The listing builds one solid part. Answer for the finished solid, in the listing's coordinates (mm). A direction names the side the tool comes from. Round coordinates to 2 decimals unless told otherwise and drop trailing zeros. Write each loop counter-clockwise with the first axis right and the second up, starting at its lowest first coordinate (ties: lowest second). Pieces come first, ordered by that corner, then holes.
Item 1: A tool of negligible diameter and unlimited length cuts with its end or side. For faces 1 (the face through (-9, -0.5, -5)), 2 (the face through (-4.06, 31.5, -4.42)), from which of +Z, -Z, +X, -X, +Y, -Y can it reach the whole face along a straight path? Write none if from no direction.
Item 2: Find section C-C on y = 7. Give the vertices of the cut face in (x, z), then the cut area to 3 significant figures.
Item 3: Find the intervals of material crossed by probe 1 along Y at (x, z) = (10.25, -8.5); probe 2 along X at (y, z) = (9, 1.5); probe 3 along Z at (x, y) = (4.75, 16), in increasing order.
Item 4: Find section A-A on z = 0. Give the vertices of the cut face in (x, y) (3 decimals), then the cut area to 3 significant figures.
Item 5: Find section B-B on x = 0. Give the vertices of the cut face in (y, z) (3 decimals).
Item 6: Find section D-D on y = 28. Give the vertices of the cut face in (x, z), then the cut area to 3 significant figures.
Item 7: Each of these flat-tipped pins is pushed along its axis until it touches: pin 1 (2 mm diameter, centred on x = -4.5, y = 2.5, fed in from -Z); pin 2 (1.5 mm diameter, centred on x = 2, y = 23.5, fed in from +Z); pin 3 (10 mm diameter, centred on y = 26.5, z = 6.5, fed in from +X); pin 4 (10 mm diameter, centred on x = 5.5, z = -1, fed in from +Y). Where does it stop, or does it pass through?
Autodesk Inventor part; units mm, degrees
ref_plane "YZ Plane" through (0, 0, 0) normal (1, 0, 0) x (0, 1, 0)
ref_plane "XZ Plane" through (0, 0, 0) normal (0, 1, 0) x (-1, 0, 0)
ref_plane "XY Plane" through (0, 0, 0) normal (0, 0, 1) x (1, 0, 0)
sketch "Skizze1" plane through (0, 0, 0) normal (1, 0, 0) x (0, 1, 0)
  line L0 (0, 13.5) -> (24, 13.5)
  line L1 (24, 13.5) -> (32, 5.5)
  line L2 (32, 5.5) -> (32, 0)
  line L3 (32, 0) -> (0, 0)
  line L4 (0, 0) -> (0, 13.5)
  arc A0 (21.85, 13.5) -> (22.85, 13.5) centre (22.35, 13.5) ccw
  line L5 (0, 0) -> (-0.5, 0)
  line L6 (-0.5, 0) -> (-0.5, 12.225)
  line L7 (-0.5, 12.225) -> (0, 12.225)
  line L8 (0, 12.225) -> (0, 0)
  line L9 (-0.5, 0) -> (-5.43, 0)
  line L10 (-5.43, 0) -> (-5.43, 10.08)
  line L11 (-5.43, 10.08) -> (-0.5, 10.08)
  line L12 (-0.5, 10.08) -> (-0.5, 0)
  point P0 (-0.5, 10.08)
  dimension "d0" = 24
  dimension "d1" = 135
  dimension "d2" = 5.5
  dimension "d3" = 1
  dimension "d4" = 0.5
  dimension "d5" = 1.15
  dimension "d6" = 0.5
  dimension "d7" = 12.225
  dimension "d8" = 4.93
  dimension "d9" = 10.08
revolve "Umdrehung1" add sketch "Skizze1" angle 360 about axis through (0, 32, 0) along (0, -1, 0) contours L0 A0 L1 L2 L3 L4 | L4 L5 L6 L7 | L9 L10 L11 L6
properties part number "00_10x_Objective_ViewSolutions_bm05073332"
Check values:
1. face 1: -Y
1. face 2: +Y
2. outline: circle Ø27 at (0, 0)
2. area: 573 mm2
3. probe 1: y = 0 to 21.89, 22.81 to 24.18
3. probe 2: x = -13.42 to 13.42
3. probe 3: z = -12.64 to 12.64
4. outline: (-13.5, 0) - (-12.225, 0) - (-12.225, -0.5) - (-10.08, -0.5) - (-10.08, -5.43) - (10.08, -5.43) - (10.08, -0.5) - (12.225, -0.5) - (12.225, 0) - (13.5, 0) - (13.5, 21.85) arc R0.5 cw to (13.5, 22.85) - (13.5, 24) - (5.5, 32) - (-5.5, 32) - (-13.5, 24) - (-13.5, 22.85) arc R0.5 cw to (-13.5, 21.85) - close
4. area: 911 mm2
5. outline: (-5.43, -10.08) - (-0.5, -10.08) - (-0.5, -12.225) - (0, -12.225) - (0, -13.5) - (21.85, -13.5) arc R0.5 cw to (22.85, -13.5) - (24, -13.5) - (32, -5.5) - (32, 5.5) - (24, 13.5) - (22.85, 13.5) arc R0.5 cw to (21.85, 13.5) - (0, 13.5) - (0, 12.225) - (-0.5, 12.225) - (-0.5, 10.08) - (-5.43, 10.08) - close
6. outline: circle Ø19 at (0, 0)
6. area: 284 mm2
7. pin 1: stops at z = -13.04
7. pin 2: stops at z = 13.44
7. pin 3: stops at x = 13.32
7. pin 4: stops at y = 32
